```python
from build123d import *

# Parameters (mm, degrees)
F0_W     = 914.4
F0_H     = 914.4
F1_DEPTH = 28.575
F3_DEPTH = 31.75
F5_D     = 3.175
F5_DEPTH = 12.7
F5_TIP   = 0.9538662327
F6_SIZE2 = 16.002
F6_SIZE  = 50.8


with BuildPart() as f1:
    # F0 (on Top) → F1 (new body)
    with BuildSketch(Plane.XY):
        Rectangle(F0_W, F0_H)
        with BuildLine():
            ThreePointArc((457.2, -457.2), (914.4, 0), (457.2, 457.2))
            Line((457.2, 457.2), (457.2, -457.2))
        make_face()
    extrude(amount=F1_DEPTH)

    # F2 (on face) → F3 (cut)
    with BuildSketch(Plane.XY.offset(28.575)):
        Polygon((330.2, -85.725), (330.2, 0), (330.2, 85.725), (279.4, 85.725), (279.4, -85.725), align=None)
    extrude(amount=-F3_DEPTH, mode=Mode.SUBTRACT)

    # F5
    with Locations(Plane(origin=(0, 0, 0), x_dir=(1, 0, 0), z_dir=(0, 0, -1))):
        with Locations((393.7, 88.9), (520.7, 88.9), (457.2, 50.8), (406.4, 0), (508, 0), (457.2, -50.8), (393.7, -88.9), (520.7, -88.9)):
            Hole(F5_D / 2, depth=F5_DEPTH)
            with Locations((0, 0, -(F5_DEPTH + F5_TIP / 2))):  # 118° drill point
                Cone(0, F5_D / 2, F5_TIP, mode=Mode.SUBTRACT)

    # F6
    f6_edges = [f1.edges().sort_by_distance(p)[0] for p in [
        (0, -457.2, 0),
        (914.4, 0, 0),
        (0, 457.2, 0),
    ]]
    f6_side = f1.faces().sort_by_distance((182.702336, 0, 0))[0]
    chamfer(f6_edges, length=F6_SIZE, length2=F6_SIZE2, reference=f6_side)


solid = f1.part
```
Source: CAD feature listing. Evaluate the final solid. Frame: model axes, mm. A direction names the side the tool comes from. Give positions to 0.01 mm unless a question says otherwise; leave off trailing zeros. Loops run counter-clockwise (first coordinate to the right, second up) from the corner with the lowest first, then second, coordinate; pieces in that order, holes last. Notation, with made-up numbers: (79.5, -10) -> (93.5, -10) arc R20 cw to (93.5, 24) -> close; hole circle Ø3 at (8.5, 76). An arc over 180 degrees is marked (long way). Use a Markdown table: item, result. Add a question column.
(1) First-contact query: pin 1 Ø1.9 at (x, y) = (520.7, 88.9) entering from -Z; pin 2 Ø6 at (y, z) = (-254, 25) entering from +X. Flat tips, straight axial feed; report the tip coordinate or a pass-through.
(2) Access query for faces 5 (the face through (279.4, 1, 14)), 6 (the face through (-6.401, -432.156, 8.113)). Directions: +Z, -Z, +X, -X, +Y, -Y. A direction counts if a zero-diameter tool reaches every point of the face in a straight line with its end or side. Return the directions, or none.
(3) Ray query, line 1 (Y direction, x = 328, z = 27.25) (3 decimals); line 2 (X direction, y = 5, z = 20.5); line 3 (X direction, y = 309.5, z = 18.75). Return the intervals inside material, ascending.
(4) Pull-direction query (Y, two-part tool) for faces 1 (the face through (305, 85.725, 14)), 2 (the face through (194, 6, 0)), 3 (the face through (6.401, 432.156, 8.113)), 4 (the face through (304, -85.725, 14)); classes: +Y half, -Y half, draft (parallel to the pull), parting line (faces both ways), or undercut.
(5) Section query A-A (z = 23.25). Output: boundary loops of the cut face in (x, y) (3 decimals).
(6) Section query B-B (x = -11). Output: boundary loops of the cut face in (y, z) (3 decimals).
Checked values:
| question | item | result |
|---|---|---|
| 1 | pin 1 | z = 13.08 |
| 1 | pin 2 | x = 839.34 |
| 2 | face 5 | +Z, -Z |
| 2 | face 6 | -Z, +X, -X, -Y |
| 3 | line 1 | -457.2 to -85.725, 85.725 to 457.2 |
| 3 | line 2 | -457.2 to 279.4, 330.2 to 914.37 |
| 3 | line 3 | -457.2 to 793.71 |
| 4 | face 1 | undercut |
| 4 | face 2 | draft |
| 4 | face 3 | +Y half |
| 4 | face 4 | undercut |
| 5 | outline | (-457.2, -457.2) -> (457.2, -457.2) arc R457.2 ccw to (457.2, 457.2) -> (-457.2, 457.2) -> close; hole (279.4, -85.725) -> (330.2, -85.725) -> (330.2, 85.725) -> (279.4, 85.725) -> close |
| 6 | outline | (-457.2, 16.002) -> (-406.4, 0) -> (406.4, 0) -> (457.2, 16.002) -> (457.2, 28.575) -> (-457.2, 28.575) -> close |
